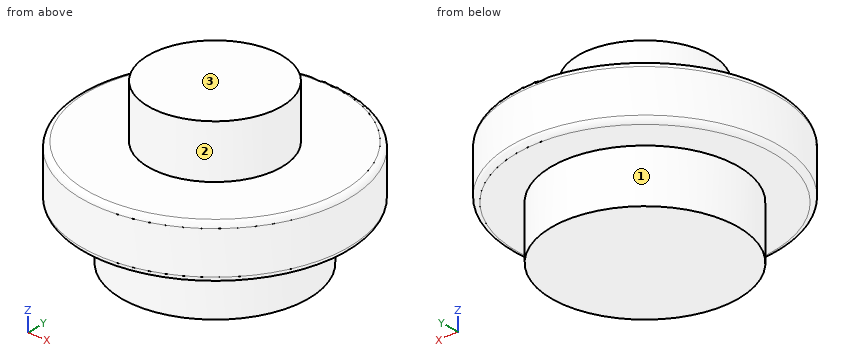
from build123d import *

# Parameters (mm, degrees)
SKETCH1_R           = 17.5
BOSS_EXTRUDE1_DEPTH = 10
SKETCH2_R           = 25
BOSS_EXTRUDE2_DEPTH = 10
SKETCH3_R           = 12.5
BOSS_EXTRUDE3_DEPTH = 10
FILLET1_R           = 1


with BuildPart() as part:
    # Sketch1 → Boss-Extrude1 (new body)
    with BuildSketch(Plane.XY):
        Circle(SKETCH1_R)
    extrude(amount=BOSS_EXTRUDE1_DEPTH)

    # Sketch2 → Boss-Extrude2 (add)
    with BuildSketch(Plane.XY.offset(10)):
        Circle(SKETCH2_R)
    extrude(amount=BOSS_EXTRUDE2_DEPTH)

    # Sketch3 → Boss-Extrude3 (add)
    with BuildSketch(Plane.XY.offset(20)):
        Circle(SKETCH3_R)
    extrude(amount=BOSS_EXTRUDE3_DEPTH)

    # Fillet1
    fillet1_edges = [part.edges().sort_by_distance(p)[0] for p in [
        (-25, 0, 10),
        (-25, 0, 20),
    ]]
    fillet(fillet1_edges, radius=FILLET1_R)


solid = part.part
Geometry: final body of the model. Coordinates: model frame, mm. Face numbers are marked on the shaded views. A direction names the side the tool comes from. Give positions to 0.01 mm unless a question says otherwise; leave off trailing zeros. Write each loop counter-clockwise with the first axis right and the second up, starting at its lowest first coordinate (ties: lowest second). Pieces come first, ordered by that corner, then holes. Notation, with made-up numbers: (62.25, 80) -> (71.25, 80) arc R24 cw to (71.25, 119) -> close; hole circle Ø9 at (86.25, 71). An arc over 180 degrees is marked (long way). Answer as a JSON object with one key per item and string values.
1. Ray query, probe 1 along Z at (x, y) = (15.5, -9); probe 2 along Z at (x, y) = (4, -15.5); probe 3 along X at (y, z) = (5, 25.75). Return the intervals inside material, ascending. Write a range as from..to.
Ans:
{"probe 1": "z = 10..20", "probe 2": "z = 0..20", "probe 3": "x = -11.46..11.46"}
2. Access query for the marked faces 1, 2 and 3. Directions: +Z, -Z, +X, -X, +Y, -Y. A direction counts if a zero-diameter tool reaches every point of the face in a straight line with its end or side. Return the directions, or none.
Ans:
{"face 1": "-Z", "face 2": "+Z", "face 3": "+Z, +X, -X, +Y, -Y"}
3. Cut plane C-C on z = 6.5. Output: boundary loops of the cut face in (x, y), and give its area (3 significant figures).
Ans:
{"outline": "circle Ø35 at (0, 0)", "area": "962 mm^2"}
4. Contact query for flat-ended pins moving along their axis: pin 1 (5 mm diameter, centred on x = 11.5, z = 13.5, fed in from -Y); pin 2 (12 mm diameter, centred on y = -17.5, z = 14.5, fed in from -X); pin 3 (6 mm diameter, centred on x = -14, z = 16.5, fed in from -Y). Output: stop coordinate, or through.
Ans:
{"pin 1": "stops at y = -23.32", "pin 2": "stops at x = -22.2", "pin 3": "stops at y = -22.45"}
5. Cut plane A-A on x = 0. Output: boundary loops of the cut face in (y, z).
Ans:
{"outline": "(-25, 11) arc R1 ccw to (-24, 10) -> (-17.5, 10) -> (-17.5, 0) -> (17.5, 0) -> (17.5, 10) -> (24, 10) arc R1 ccw to (25, 11) -> (25, 19) arc R1 ccw to (24, 20) -> (12.5, 20) -> (12.5, 30) -> (-12.5, 30) -> (-12.5, 20) -> (-24, 20) arc R1 ccw to (-25, 19) -> close"}
6. Cut plane D-D on z = 23.75. Output: boundary loops of the cut face in (x, y), and give its area (3 significant figures).
Ans:
{"outline": "circle Ø25 at (0, 0)", "area": "491 mm^2"}
